Source: CAD feature listing. Evaluate the final solid. Frame: model axes, mm. Give positions to 0.01 mm unless a question says otherwise; leave off trailing zeros. Loops run counter-clockwise (first coordinate to the right, second up) from the corner with the lowest first, then second, coordinate; pieces in that order, holes last. Notation, with made-up numbers: (33, -28.5) -> (73, -28.5) arc R30 ccw to (73, -3.5) -> close; hole circle Ø9 at (32.25, -19). An arc over 180 degrees is marked (long way). Answer as a JSON object with one key per item and string values. Group by question number.
Autodesk Inventor part; units mm, degrees
ref_plane "YZ Plane" through (0, 0, 0) normal (1, 0, 0) x (0, 1, 0)
ref_plane "XZ Plane" through (0, 0, 0) normal (0, 1, 0) x (-1, 0, 0)
ref_plane "XY Plane" through (0, 0, 0) normal (0, 0, 1) x (1, 0, 0)
sketch "Sketch1" plane through (0, 0, 0) normal (0, 1, 0) x (-1, 0, 0)
  line L0 (480.5, 1604) -> (474.5, 1604)
  line L1 (474.5, 1604) -> (474.5, 0)
  line L2 (474.5, 0) -> (480.5, 0)
  line L3 (480.5, 0) -> (480.5, 1604)
  line L4 (0, 0) -> (0, 1673.0415)
  point P0 (477.5, 0)
  dimension "d0" = 6
  dimension "d1" = 1604
  dimension "d2" = 949
revolve "Revolution1" add sketch "Sketch1" angle 359.9 about axis through (0, 0, 0) along (0, 0, 1)
sketch "Sketch2" plane through (0, 0, 0) normal (0, 1, 0) x (-1, 0, 0)
  circle A0 centre (0, 1109) radius 207
  circle A1 centre (0, 215) radius 40
  circle A2 centre (0, 1499) radius 40
  line L0 (474.5, 1604) -> (-474.5, 1604)
  point P0 (0, 0)
  point P1 (474.4993, 1604)
  dimension "d4" = 414
  dimension "d5" = 80
  dimension "d6" = 80
  dimension "d7" = 215
  dimension "d8" = 105
  dimension "d9" = 495
extrude "Extrusion1" cut sketch "Sketch2" against normal through all
equation "\"d1\" = Высота_сред_части"
equation "\"d2\" = Внутр_Диам"
equation "\"d4\" = Внутр_диам_ревиз_окна"
equation "\"d5\" = Внешний_диам_трубы_подкл"
equation "\"d6\" = Внешний_диам_трубы_подкл"
equation "\"BendRadius\" = Thickness"
equation "\"BendReliefWidth\" = Thickness"
equation "\"BendReliefDepth\" = 0.5 * Thickness"
equation "\"CornerReliefSize\" = 4 * Thickness"
equation "\"MinimumRemnant\" = 2 * Thickness"
equation "\"TransitionRadius\" = BendRadius"
equation "\"JacobiRadiusSize\" = BendRadius"
equation "\"GapSize\" = Thickness"
properties part number "Стенка фильтра D1000"
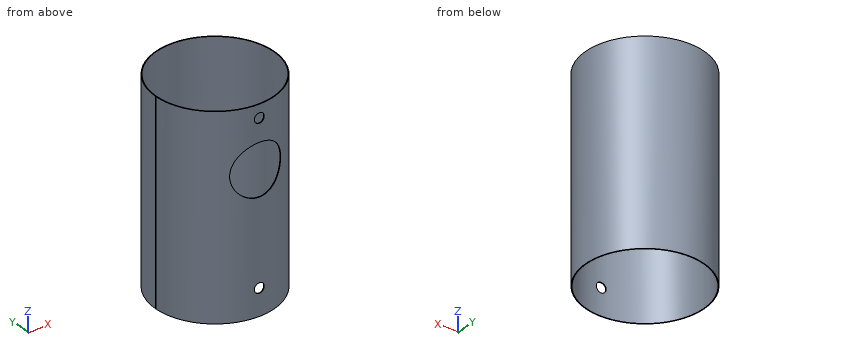
(1) Section query D-D on z = 215. Return the cut outline in (x, y), plus the area to 3 significant figures.
(2) Section query A-A on x = 0. Return the cut outline in (y, z).
(3) First-contact query: pin 1 (8 mm diameter, centred on x = 138, z = 937, fed in from +Y); pin 2 (12 mm diameter, centred on x = 71.5, z = 309.5, fed in from -Y); pin 3 (2 mm diameter, centred on x = -327, z = 1237, fed in from -Y). Flat tips, straight axial feed; report the tip coordinate or a pass-through.
(4) Material intervals for line 1 (Z direction, x = 0, y = -475.5); line 2 (Y direction, x = 0, z = 721), sorted ascending. Write a range as from..to.
(5) Section query B-B on y = -158. Return the cut outline in (x, z), plus the area to 3 significant figures.
(6) Section query C-C on x = -159. Return the cut outline in (y, z), plus the area to 3 significant figures.
Result:
{
 "1": {"outline": "(-480.5, 0) arc R480.5 ccw to (-40, -478.83) -> (-40, -472.81) arc R474.5 cw to (-474.5, 0) -> close; (-480.5, 0.84) -> (-474.5, 0.83) arc R474.5 cw (long way) to (40, -472.81) -> (40, -478.83) arc R480.5 ccw (long way) to start", "area": "17,500 mm²"},
 "2": {"outline": "(-480.5, 0) -> (-474.5, 0) -> (-474.5, 175) -> (-480.5, 175) -> close; (-480.5, 255) -> (-474.5, 255) -> (-474.5, 902) -> (-480.5, 902) -> close; (-480.5, 1316) -> (-474.5, 1316) -> (-474.5, 1459) -> (-480.5, 1459) -> close; (-480.5, 1539) -> (-474.5, 1539) -> (-474.5, 1604) -> (-480.5, 1604) -> close; (474.5, 0) -> (480.5, 0) -> (480.5, 1604) -> (474.5, 1604) -> close"},
 "3": {"pin 1": "y = 461.44", "pin 2": "y = -476.01", "pin 3": "y = -352.99"},
 "4": {"line 1": "0..175, 255..902, 1316..1459, 1539..1604", "line 2": "-480.5..-474.5, 474.5..480.5"},
 "5": {"outline": "(-453.78, 0) -> (-447.42, 0) -> (-447.42, 1604) -> (-453.78, 1604) -> close; (447.42, 0) -> (453.78, 0) -> (453.78, 1604) -> (447.42, 1604) -> close", "area": "20,400 mm²"},
 "6": {"outline": "(-453.43, 0) -> (-447.07, 0) -> (-447.07, 976.46) -> (-453.43, 976.46) -> close; (-453.43, 1241.54) -> (-447.07, 1241.54) -> (-447.07, 1604) -> (-453.43, 1604) -> close; (447.07, 0) -> (453.43, 0) -> (453.43, 1604) -> (447.07, 1604) -> close", "area": "18,700 mm²"}
}
